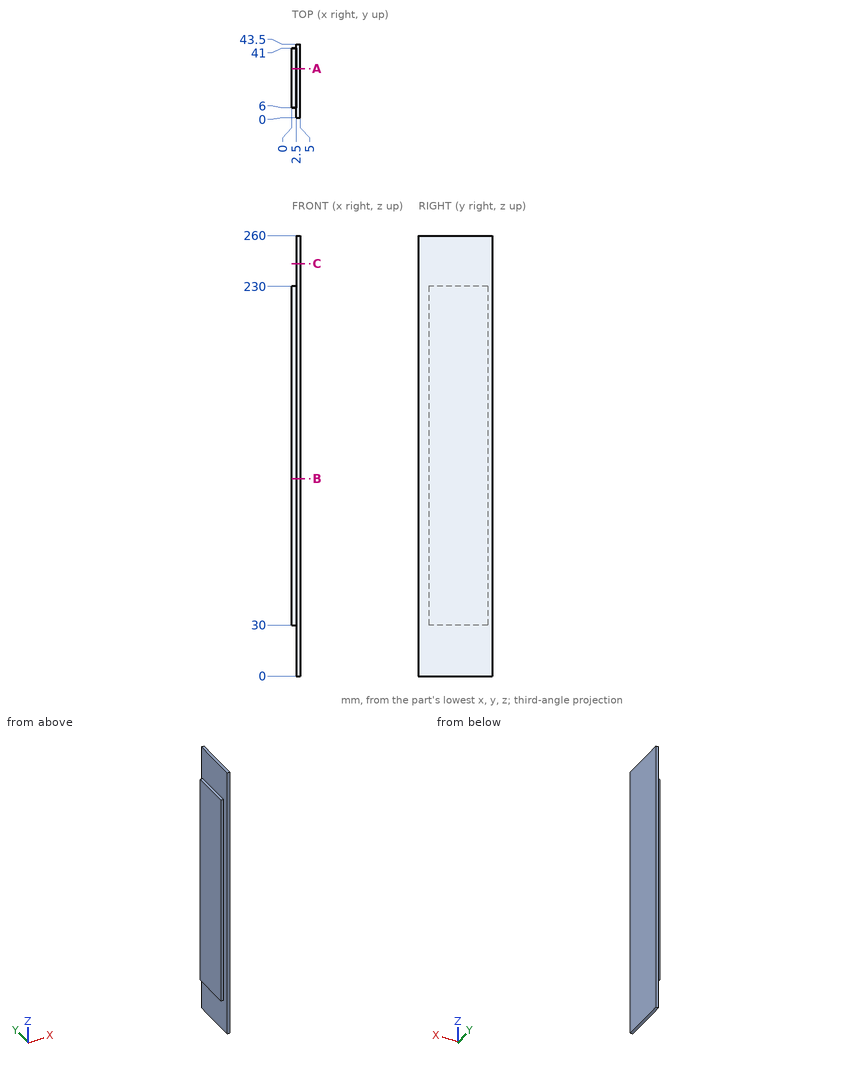
Input: dimensioned drawing with shaded views. Units: mm. Origin: part minimum x, y, z. Round coordinates to 2 decimals unless told otherwise and drop trailing zeros. Order: outer loops, then holes, each group sorted by start corner. A loop starts at its lowest first (then second) coordinate and runs counter-clockwise, first axis right, second up.
Q1. Section A-A, the plane y = 29. Output: boundary loops of the cut face in (x, z).
Result sheet:
outline: (0, 30) - (2.5, 30) - (2.5, 0) - (5, 0) - (5, 260) - (2.5, 260) - (2.5, 230) - (0, 230) - close
Q2. Section C-C, the plane z = 243.5. Output: boundary loops of the cut face in (x, y), and give its area (3 significant figures).
Result sheet:
outline: (2.5, 0) - (5, 0) - (5, 43.5) - (2.5, 43.5) - close
area: 109 mm2
Q3. Material intervals for probe 1 along Z at (x, y) = (1.3, 17.5); probe 2 along Y at (x, z) = (2.3, 215); probe 3 along X at (y, z) = (12, 28), sorted ascending.
Result sheet:
probe 1: z = 30 to 230
probe 2: y = 6 to 41
probe 3: x = 2.5 to 5
Q4. Pin query (flat end, axial travel): pin 1 (2 mm diameter, centred on x = 1, y = 27, fed in from -Z); pin 2 (1.2 mm diameter, centred on x = 1, z = 121.5, fed in from +Y); pin 3 (2 mm diameter, centred on x = 0.5, z = 81, fed in from -Y). Return the tip coordinate at first contact, or that it passes through.
Result sheet:
pin 1: stops at z = 30
pin 2: stops at y = 41
pin 3: stops at y = 6
Q5. Section B-B, the plane z = 116.5. Output: boundary loops of the cut face in (x, y), and give its area (3 significant figures).
Result sheet:
outline: (0, 6) - (2.5, 6) - (2.5, 0) - (5, 0) - (5, 43.5) - (2.5, 43.5) - (2.5, 41) - (0, 41) - close
area: 196 mm2
